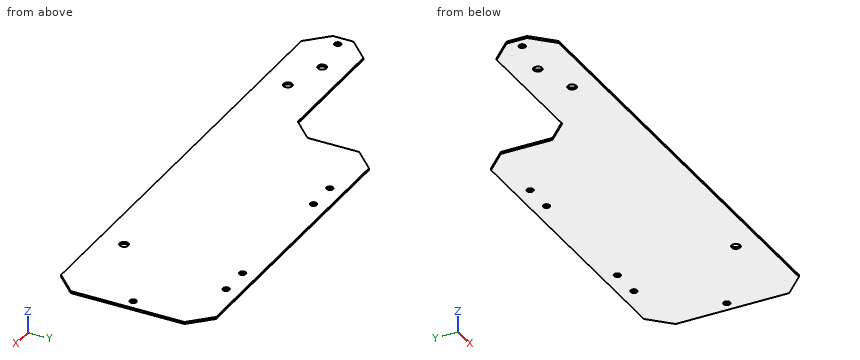
from build123d import *

# Parameters (mm, degrees)
SKETCH_1_W          = 240
SKETCH_1_H          = 75
EXTRUDE_1_DEPTH     = 1
SKETCH_4_W          = 80
SKETCH_4_H          = 45
CUT_EXTRUDE_3_DEPTH = 10
CHAMFER_1_SIZE      = 10
SKETCH_5_R          = 1.6
SKETCH_5_R_2        = 2.1
CUT_EXTRUDE_4_DEPTH = 10


with BuildPart() as part:
    # 草图1 → 凸台-拉伸1 (new body)
    with BuildSketch(Plane.XY):
        with Locations((120, 37.5)):
            Rectangle(SKETCH_1_W, SKETCH_1_H)
    extrude(amount=EXTRUDE_1_DEPTH)

    # 草图4 → 切除-拉伸3 (cut)
    with BuildSketch(Plane(origin=(0, 0, 0), x_dir=(-1, 0, 0), z_dir=(0, 0, -1))):
        with Locations((-40, 52.5)):
            Rectangle(SKETCH_4_W, SKETCH_4_H)
    extrude(amount=-CUT_EXTRUDE_3_DEPTH, mode=Mode.SUBTRACT)

    # 倒角1
    chamfer_1_edges = [part.edges().sort_by_distance(p)[0] for p in [
        (80, 75, 0.5),
        (0, 30, 0.5),
        (80, 30, 0.5),
        (240, 75, 0.5),
        (240, 0, 0.5),
        (0, 0, 0.5),
    ]]
    chamfer(chamfer_1_edges, length=CHAMFER_1_SIZE)

    # 草图5 → 切除-拉伸4 (cut)
    with BuildSketch(Plane(origin=(0, 0, 0), x_dir=(-1, 0, 0), z_dir=(0, 0, -1))):
        with Locations((-5, 15)):
            Circle(SKETCH_5_R)
        with Locations((-195, 12)):
            Circle(SKETCH_5_R_2)
        with Locations((-45, 12)):
            Circle(SKETCH_5_R_2)
        with Locations((-235, 37.5)):
            Circle(SKETCH_5_R)
        with Locations((-207.5, 68)):
            Circle(SKETCH_5_R)
        with Locations((-192.5, 68)):
            Circle(SKETCH_5_R)
        with Locations((-127.5, 68)):
            Circle(SKETCH_5_R)
        with Locations((-112.5, 68)):
            Circle(SKETCH_5_R)
        with Locations((-25, 18)):
            Circle(SKETCH_5_R_2)
    extrude(amount=-CUT_EXTRUDE_4_DEPTH, mode=Mode.SUBTRACT)


solid = part.part
Check sheet for the modelled part. Datum: model origin and axes. Units: mm. Round coordinates to 2 decimals unless told otherwise and drop trailing zeros. Loops run counter-clockwise (first coordinate to the right, second up) from the corner with the lowest first, then second, coordinate; pieces in that order, holes last. Notation, with made-up numbers: M 20,57.5 L 53,57.5 A35 cw 53,90.5 Z; hole C 87.25,7 d11. An arc over 180 degrees is marked long. One line per item, written item: value.
(1) Sectioned sample at A-A, the plane x = 45. Record the cut outline in (y, z).
Computed values:
outline: M 0,0 L 9.9,0 L 9.9,1 L 0,1 Z; M 14.1,0 L 30,0 L 30,1 L 14.1,1 Z
(2) Thickness scan on line 1 (X direction, y = 68, z = 0.7); line 2 (Y direction, x = 112.5, z = 0.6); line 3 (Y direction, x = 45, z = 0.2). Record the ranges inside material, lowest first.
Computed values:
line 1: x = 83 to 110.9, 114.1 to 125.9, 129.1 to 190.9, 194.1 to 205.9, 209.1 to 237
line 2: y = 0 to 66.4, 69.6 to 75
line 3: y = 0 to 9.9, 14.1 to 30
(3) Sectioned sample at C-C, the plane y = 54. Record the cut outline in (x, z), then the cut area to 3 significant figures.
Computed values:
outline: M 80,0 L 240,0 L 240,1 L 80,1 Z
area: 160 mm^2
(4) Sectioned sample at B-B, the plane z = 0.6. Count the separate pieces of the cut face and the enclosed holes in it, then the cut area to 3 significant figures.
Computed values:
separate pieces: 1
enclosed holes: 9
area: 14,100 mm^2
